Build history of the part. All positions in model axes, mm. A direction names the side the tool comes from. Coordinates: 2 decimals unless noted, no trailing zeros. Loops run counter-clockwise (first coordinate to the right, second up) from the corner with the lowest first, then second, coordinate; pieces in that order, holes last.
(1) Slice it at B-B (y = -72). Give the cut face in (x, z), and give its area (3 significant figures).
(2) Wall check: L1, parallel to Y at x = 0, z = 0.4; L2, parallel to Y at x = 1, z = 1.35; L3, parallel to Y at x = 53.5, z = 0.1. Give the ranges that are in metal, low to high.
(3) Slice it at A-A (z = 0.5). Give the number of separate pieces and of enclosed holes in the cut face, and give its area (3 significant figures).
(4) Slice it at C-C (x = 44.5). Give the cut face in (y, z).
(5) Two-plate mould, pull along X, no slides. Class faces 3 (the face through (78.386, -66.698, 0.783)), 4 (the face through (-3.959, -75.525, 0.783)), 5 (the face through (-0.45, -81.93, 0.78)), 6 (the face through (38.9, -92.72, 0.78)): pulls with the +X half, pulls with the -X half, needs draft (parallel to the pull), parting line crosses it, or undercut.
(6) Tool access for faces 1 (the face through (-3.915, -13.424, 0.783)), 2 (the face through (39, -47, 0)): list every direction of +Z, -Z, +X, -X, +Y, -Y with a clear straight run to the whole face (end or side of a thin tool).
Autodesk Inventor part; units mm, degrees
ref_plane "YZ Plane" through (0, 0, 0) normal (1, 0, 0) x (0, 1, 0)
ref_plane "XZ Plane" through (0, 0, 0) normal (0, 1, 0) x (-1, 0, 0)
ref_plane "XY Plane" through (0, 0, 0) normal (0, 0, 1) x (1, 0, 0)
sketch "main" plane through (0, 0, 0) normal (0, 0, 1) x (1, 0, 0)
  line L0 (57.2021, -70.0851) -> (14.0558, -70.0851)
  line L1 (5.3685, -68.5533) -> (-23.0916, -58.1947)
  line L2 (-26.2252, -53.7194) -> (-26.2252, -47.3776)
  arc A0 (-23.3526, -44.217) -> (-23.3526, 15.8337) centre (-26.2252, -14.1917) ccw
  line L3 (-26.2252, 18.9943) -> (-26.2252, 30.2583)
  line L4 (-21.4627, 35.0208) -> (10.7437, 35.0208)
  line L5 (13.1667, 33.8976) -> (49.3481, -8.8317)
  arc A1 (-21.4627, 35.0208) -> (-26.2252, 30.2583) centre (-21.4627, 30.2583) ccw
  circle A2 centre (-21.4627, 30.2583) radius 2.0955
  arc A3 (-26.2252, 18.9943) -> (-23.3526, 15.8337) centre (-23.0502, 18.9943) ccw
  arc A4 (-23.3526, -44.217) -> (-26.2252, -47.3776) centre (-23.0502, -47.3776) ccw
  arc A5 (-26.2252, -53.7194) -> (-23.0916, -58.1947) centre (-21.4627, -53.7194) ccw
  circle A6 centre (-21.4627, -53.7194) radius 2.0955
  arc A7 (13.1667, 33.8976) -> (10.7437, 35.0208) centre (10.7437, 31.8458) ccw
  circle A8 centre (57.2021, -63.7351) radius 2.0955
  arc A9 (50.6625, -11.395) -> (49.3481, -8.8317) centre (44.5021, -12.9351) ccw
  circle A10 centre (44.5021, -12.9351) radius 2.0955
  line L6 (50.6625, -11.395) -> (63.3625, -62.195)
  arc A11 (57.2021, -70.0851) -> (63.3625, -62.195) centre (57.2021, -63.7351) ccw
  circle A12 centre (19.1021, -63.7351) radius 2.0955
  arc A13 (5.3685, -68.5533) -> (14.0558, -70.0851) centre (14.0558, -44.6851) ccw
  point P0 (-12.3105, 3.8443)
  point P1 (9.5771, -70.0851)
  point P2 (-26.2252, -57.0542)
  point P3 (-26.2252, -44.3542)
  point P4 (-26.2252, 15.9708)
  point P5 (-26.2252, 35.0208)
  point P6 (20.6896, -70.0851)
  dimension "d14" = 38.1
  dimension "d15" = 160
  dimension "d16" = 12.7
  dimension "d17" = 19.05
  dimension "d18" = 4.7625
  dimension "d19" = 4.191
  dimension "d20" = 3.175
  dimension "d21" = 4.7625
  dimension "d22" = 4.191
  dimension "d23" = 4.191
  dimension "d24" = 4.191
  dimension "d25" = 4.191
  dimension "d26" = 25.4
sketch "Sketch1" plane through (0, 0, 0) normal (0, 0, 1) x (1, 0, 0)
  line L0 (78.6648, -100.3435) -> (35.5185, -100.3435)
  line L1 (26.8312, -98.8117) -> (-1.6289, -88.453)
  line L2 (-4.7625, -83.9778) -> (-4.7625, -77.636)
  arc A0 (-1.8899, -74.4754) -> (-1.8899, -14.4246) centre (-4.7625, -44.45) ccw
  line L3 (-4.7625, -11.264) -> (-4.7625, 0)
  line L4 (0, 4.7625) -> (32.2064, 4.7625)
  line L5 (34.6294, 3.6392) -> (70.8108, -39.09)
  arc A1 (0, 4.7625) -> (-4.7625, 0) centre (0, 0) ccw
  circle A2 centre (0, 0) radius 2.0955
  arc A3 (-4.7625, -11.264) -> (-1.8899, -14.4246) centre (-1.5875, -11.264) ccw
  arc A4 (-1.8899, -74.4754) -> (-4.7625, -77.636) centre (-1.5875, -77.636) ccw
  arc A5 (-4.7625, -83.9778) -> (-1.6289, -88.453) centre (0, -83.9778) ccw
  circle A6 centre (0, -83.9778) radius 2.0955
  arc A7 (34.6294, 3.6392) -> (32.2064, 4.7625) centre (32.2064, 1.5875) ccw
  circle A8 centre (78.6648, -93.9935) radius 2.0955
  arc A9 (72.1252, -41.6534) -> (70.8108, -39.09) centre (65.9648, -43.1935) ccw
  circle A10 centre (65.9648, -43.1935) radius 2.0955
  line L6 (72.1252, -41.6534) -> (84.8252, -92.4534)
  arc A11 (78.6648, -100.3435) -> (84.8252, -92.4534) centre (78.6648, -93.9935) ccw
  circle A12 centre (40.5648, -93.9935) radius 2.0955
  arc A13 (26.8312, -98.8117) -> (35.5185, -100.3435) centre (35.5185, -74.9435) ccw
extrude "Extrusion1" add sketch "Sketch1" along normal blind 1.5875
properties part number "hang_gusset" material "Acetal Resin, White"
Response values:
1. outline: (7.52, 0) - (79.71, 0) - (79.71, 1.59) - (7.52, 1.59) - close
1. area: 115 mm2
2. L1: y = -89.05 to -86.07, -81.88 to -74.23, -14.67 to -2.1, 2.1 to 4.76
2. L2: y = -89.41 to -85.82, -82.14 to -74.06, -14.84 to -1.84, 1.84 to 4.76
2. L3: y = -100.34 to -18.65
3. separate pieces: 1
3. enclosed holes: 5
3. area: 5,880 mm2
4. outline: (-100.34, 0) - (-8.02, 0) - (-8.02, 1.59) - (-100.34, 1.59) - close
5. face 3: pulls with the +X half
5. face 4: pulls with the -X half
5. face 5: undercut
5. face 6: undercut
6. face 1: +Z, -Z, -X
6. face 2: -Z, +X, -X, +Y, -Y
